from build123d import *

# Parameters (mm, degrees)
F0_W          = 101.6
F0_H          = 50.8
F1_DEPTH      = 101.6
F3_DEPTH      = 50.801
F4_W          = 50.8
F4_H          = 76.2
F5_DEPTH      = 50.8
F6_R          = 38.1
F6_R_2        = 25.4
F7_DEPTH      = 25.4
F7_DEPTH_BACK = 76.2
F8_DEPTH      = 76.201


with BuildPart() as f1:
    # F0 (on Top) → F1 (new body)
    with BuildSketch(Plane.XY):
        with Locations((-50.8, 25.4)):
            Rectangle(F0_W, F0_H)
    extrude(amount=F1_DEPTH)

    # F2 (on face) → F3 (cut, through all)
    with BuildSketch(Plane(origin=(0, 50.8, 0), x_dir=(-1, 0, 0), z_dir=(0, 1, 0))):
        Polygon((0, 76.2), (25.4, 101.6), (0, 101.6), align=None)
        Polygon((101.6, 101.6), (76.2, 101.6), (101.6, 76.2), align=None)
    extrude(amount=-F3_DEPTH, mode=Mode.SUBTRACT)

    # F4 (on face) → F5 (join)
    with BuildSketch(Plane(origin=(0, 50.8, 0), x_dir=(-1, 0, 0), z_dir=(0, 1, 0))):
        with Locations((50.8, 38.1)):
            Rectangle(F4_W, F4_H)
    extrude(amount=F5_DEPTH)

    # F6 (on face) → F7 (join, two sides)
    with BuildSketch(Plane(origin=(-76.2, 0, 0), x_dir=(0, -1, 0), z_dir=(-1, 0, 0))) as f7_sk:
        with Locations((-101.6, 38.1)):
            Circle(F6_R)
        with Locations((-101.6, 38.1)):
            Circle(F6_R_2, mode=Mode.SUBTRACT)
    extrude(amount=F7_DEPTH)
    extrude(f7_sk.sketch, amount=-F7_DEPTH_BACK)

    # F7_face (on face) → F8 (cut, through all)
    with BuildSketch(Plane(origin=(-76.2, 90.819905, 38.1), x_dir=(0, -1, 0), z_dir=(-1, 0, 0))):
        with BuildLine():
            ThreePointArc((-10.780095, -25.4), (7.180417, -17.960512), (14.619905, 0))
            ThreePointArc((14.619905, 0), (7.180417, 17.960512), (-10.780095, 25.4))
            Line((-10.780095, 25.4), (-10.780095, -25.4))
        make_face()
    extrude(amount=-F8_DEPTH, mode=Mode.SUBTRACT)


solid = f1.part
Source: CAD feature listing. Evaluate the final solid. Frame: model axes, mm. A direction names the side the tool comes from. Round coordinates to 2 decimals unless told otherwise and drop trailing zeros. Order: outer loops, then holes, each group sorted by start corner. A loop starts at its lowest first (then second) coordinate and runs counter-clockwise, first axis right, second up. Notation, with made-up numbers: (6.25, 64.25) - (57.25, 64.25) arc R20 cw to (57.25, 85.25) - close; hole circle Ø11 at (48, 43). An arc over 180 degrees is marked (long way). Use a Markdown table: item, result. Add a question column.
1. First-contact query: pin 1 (2 mm diameter, centred on x = -80.5, y = 77.5, fed in from +Z); pin 2 (1.5 mm diameter, centred on x = -31.5, z = 73.5, fed in from +Y); pin 3 (1.5 mm diameter, centred on x = -91, y = 121, fed in from +Z). Flat tips, straight axial feed; report the tip coordinate or a pass-through.
2. Set-up query: faces 4 (the flat face through (0, 94, 13)), 5 (the flat face through (-50, 76, 76.2)), 6 (the flat face through (-52, 50.8, 84)), 7 (the flat face through (-76.2, 59, 38)), 8 (the flat face through (-101.6, 25, 38)). Return all of +Z, -Z, +X, -X, +Y, -Y with unobstructed straight access to the full face (end or side cutting, diameter ignored); none if empty.
3. Section query B-B (y = 117). Return the cut outline in (x, z).
4. Mould query, pull axis Y, two halves, no side actions, for faces 1 (the flat face through (-25.4, 59, 38)), 2 (the flat face through (-88.7, 25.8, 89.1)), 3 (the flat face through (-52, 0, 50)). Classes: +Y half, -Y half, draft (parallel to the pull), parting line (faces both ways), or undercut.
5. Section query D-D (x = -34). Return the cut outline in (y, z), then the cut area to 3 significant figures.
6. Line query: probe 1 along Y at (x, z) = (-93, 38.1); probe 2 along Z at (x, y) = (-82, 101); probe 3 along Y at (x, z) = (-91, 26). Output: solid intervals per line, ascending.
7. Section query C-C (z = 53). Return the cut outline in (x, y).
8. Section query A-A (x = -16). Return the cut outline in (y, z), then the cut area to 3 significant figures.
Derived:
| question | item | result |
|---|---|---|
| 1 | pin 1 | z = 68.4 |
| 1 | pin 2 | y = 117.44 |
| 1 | pin 3 | z = 71.32 |
| 2 | face 4 | +Z, -Z, +X, +Y, -Y |
| 2 | face 5 | +Z, +X, -X, +Y |
| 2 | face 6 | +Z |
| 2 | face 7 | -X |
| 2 | face 8 | +Z, -Z, -X, +Y, -Y |
| 3 | outline | (-101.6, 3.25) - (0, 3.25) - (0, 17.9) - (-101.6, 17.9) - close; (-101.6, 58.3) - (0, 58.3) - (0, 72.95) - (-101.6, 72.95) - close |
| 4 | face 1 | undercut |
| 4 | face 2 | draft |
| 4 | face 3 | -Y half |
| 5 | outline | (0, 0) - (101.6, 0) arc R38.1 ccw to (101.6, 76.2) - (50.8, 76.2) - (50.8, 101.6) - (0, 101.6) - close; hole (76.2, 38.1) arc R25.4 ccw to (101.6, 12.7) arc R25.4 ccw (long way) to start |
| 5 | area | 9,290 mm2 |
| 6 | probe 1 | 0 to 50.8, 63.5 to 76.2, 127 to 139.7 |
| 6 | probe 2 | 0 to 12.71, 63.49 to 76.2 |
| 6 | probe 3 | 0 to 50.8, 65.47 to 79.27, 123.93 to 137.73 |
| 7 | outline | (-101.6, 0) - (0, 0) - (0, 50.8) - (-25.4, 50.8) - (-25.4, 66.53) - (0, 66.53) - (0, 81.03) - (-101.6, 81.03) - (-101.6, 66.53) - (-76.2, 66.53) - (-76.2, 50.8) - (-101.6, 50.8) - close; (-101.6, 122.17) - (0, 122.17) - (0, 136.67) - (-101.6, 136.67) - close |
| 8 | outline | (0, 0) - (50.8, 0) - (50.8, 92.2) - (0, 92.2) - close; circle Ø76.2 at (101.6, 38.1); hole circle Ø50.8 at (101.6, 38.1) |
| 8 | area | 7,220 mm2 |
